Read the model definition and answer for the solid it produces. Units are mm, in the model's axes. Face numbers are marked on the shaded views. A direction names the side the tool comes from. Coordinates: 2 decimals unless noted, no trailing zeros. Write each loop counter-clockwise with the first axis right and the second up, starting at its lowest first coordinate (ties: lowest second). Pieces come first, ordered by that corner, then holes.
(1) Section B-B on x = -95.5 is taken. Write down the section's boundary in (y, z).
(2) Section C-C on z = 10.75 is taken. Write down the section's boundary in (x, y), then the cut area to 3 significant figures.
(3) The mould has two halves that part along Y. Classify the marked faces 1, 2 and 3: +Y half, -Y half, draft (parallel to the pull), parting line (faces both ways), or undercut.
(4) Given pin 1 (4 mm diameter, centred on x = 66.5, y = -72, fed in from -Z); pin 2 (6 mm diameter, centred on x = 46, z = 14, fed in from +Y); pin 3 (7.5 mm diameter, centred on x = 3, z = 12.5, fed in from +Y), each flat-ended and moving along its own axis, determine where each tip first touches the part or whether it passes through.
(5) Find the intervals of material crossed by probe 1 along X at (y, z) = (-64.5, 16.75); probe 2 along Y at (x, z) = (97, 3.25); probe 3 along X at (y, z) = (-3, 11.5), in increasing order.
(6) Section A-A on y = -94 is taken. Write down the section's boundary in (x, z), then the cut area to 3 significant figures.
(7) Which of the six approach directions +Z, -Z, +X, -X, +Y, -Y give full straight-line access (tool end or side, diameter ignored) to the marked faces 4, 5 and 6?
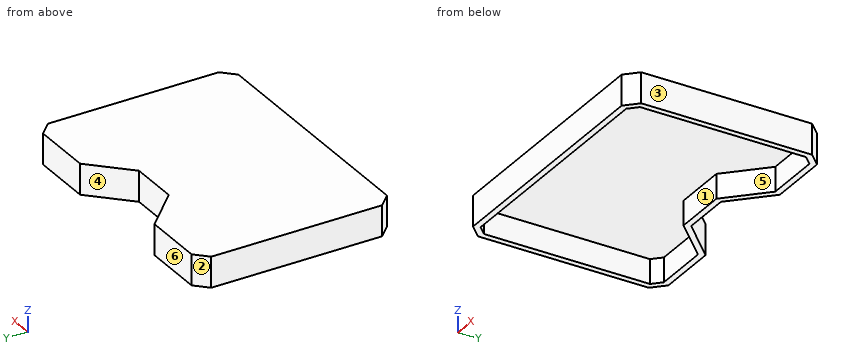
Solid Edge part; units mm, degrees
sketch "Sketch1" plane through (0, 0, 0) normal (0, 0, 1) x (1, 0, 0)
  line L0 (-110, 19.1949) -> (-110, -120.8051)
  line L1 (-110, -120.8051) -> (-100, -130.8051)
  line L2 (-100, -130.8051) -> (100, -130.8051)
  line L3 (100, -130.8051) -> (110, -120.8051)
  line L4 (110, -120.8051) -> (110, 19.1949)
  line L5 (110, 19.1949) -> (100, 29.1949)
  line L6 (100, 29.1949) -> (50, 29.1949)
  line L7 (50, 29.1949) -> (20, -0.8051)
  line L8 (20, -0.8051) -> (-20, -0.8051)
  line L9 (-20, -0.8051) -> (-50, 29.1949)
  line L10 (-50, 29.1949) -> (-100, 29.1949)
  line L11 (-100, 29.1949) -> (-110, 19.1949)
  dimension "D1" = 50
extrude "Body_ThinWallOptions" add sketch "Sketch1" along normal blind 25
shell "Inside" thickness 5 removed faces 1 at (-75.5333, -102.5384, 0)
Response:
1. outline: (-130.81, 0) - (-125.81, 0) - (-125.81, 20) - (24.19, 20) - (24.19, 0) - (29.19, 0) - (29.19, 25) - (-130.81, 25) - close
2. outline: (-110, -120.81) - (-100, -130.81) - (100, -130.81) - (110, -120.81) - (110, 19.19) - (100, 29.19) - (50, 29.19) - (20, -0.81) - (-20, -0.81) - (-50, 29.19) - (-100, 29.19) - (-110, 19.19) - close; hole (-105, -118.73) - (-97.93, -125.81) - (97.93, -125.81) - (105, -118.73) - (105, 17.12) - (97.93, 24.19) - (52.07, 24.19) - (22.07, -5.81) - (-22.07, -5.81) - (-52.07, 24.19) - (-97.93, 24.19) - (-105, 17.12) - close
2. area: 3,720 mm2
3. face 1: undercut
3. face 2: +Y half
3. face 3: draft
4. pin 1: stops at z = 20
4. pin 2: stops at y = 28.19
4. pin 3: stops at y = -0.81
5. probe 1: x = -110 to -105, 105 to 110
5. probe 2: y = -130.81 to -125.81, 24.19 to 29.19
5. probe 3: x = -110 to -105, -24.88 to 24.88, 105 to 110
6. outline: (-110, 0) - (-105, 0) - (-105, 20) - (105, 20) - (105, 0) - (110, 0) - (110, 25) - (-110, 25) - close
6. area: 1,300 mm2
7. face 4: +Z, -Z, +Y
7. face 5: -Z
7. face 6: +Z, -Z, +X, -X, +Y
